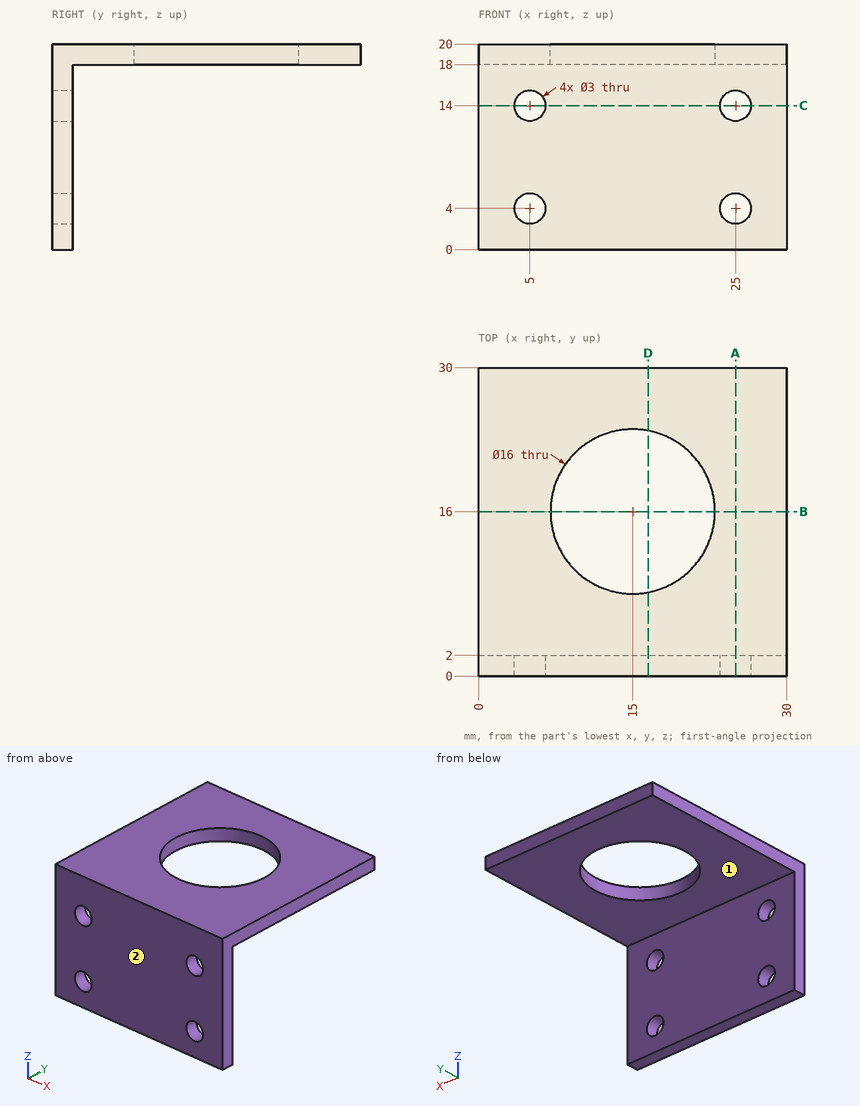
Verification items for this drawing (mm, ordinates from the low corner). A direction names the side the tool comes from. Round coordinates to 2 decimals unless told otherwise and drop trailing zeros. Write each loop counter-clockwise with the first axis right and the second up, starting at its lowest first coordinate (ties: lowest second). Pieces come first, ordered by that corner, then holes. Notation, with made-up numbers: (43.5, -4.75) - (59.5, -4.75) arc R28 ccw to (59.5, 21.25) - close; hole circle Ø4 at (22, 62). An arc over 180 degrees is marked (long way). Answer as a JSON object with one key per item and string values. Group by question number.
Q1. Section check C-C, the plane z = 14. Enter the section's corners in (x, y).
Q2. Section check A-A, the plane x = 25. Enter the section's corners in (y, z), plus the area to 3 significant figures.
Q3. Thickness scan on line 1 (X direction, y = 0.7, z = 4); line 2 (Y direction, x = 24.5, z = 2); line 3 (Z direction, x = 5.25, y = 20). Record the ranges inside material, lowest first.
Q4. Section check D-D, the plane x = 16.5. Enter the section's corners in (y, z).
Q5. Tool access check on the marked faces 1 and 2. Record the directions out of +Z, -Z, +X, -X, +Y, -Y that give a thin tool (end or side, any length) a straight path to the whole face; none if there is none.
Q6. Section check B-B, the plane y = 16. Enter the section's corners in (x, z), plus the area to 3 significant figures.
Q7. Go/stop test with flat-tipped pins: pin 1 Ø14 at (x, y) = (10, 22) entering from -Z; pin 2 Ø5 at (x, z) = (5, 14) entering from +Y. Record where each tip stops, or that it passes through.
Found:
{
 "1": {"outline": "(0, 0) - (3.5, 0) - (3.5, 2) - (0, 2) - close; (6.5, 0) - (23.5, 0) - (23.5, 2) - (6.5, 2) - close; (26.5, 0) - (30, 0) - (30, 2) - (26.5, 2) - close"},
 "2": {"outline": "(0, 0) - (2, 0) - (2, 2.5) - (0, 2.5) - close; (0, 5.5) - (2, 5.5) - (2, 12.5) - (0, 12.5) - close; (0, 15.5) - (2, 15.5) - (2, 18) - (30, 18) - (30, 20) - (0, 20) - close", "area": "84.0 mm^2"},
 "3": {"line 1": "x = 0 to 3.5, 6.5 to 23.5, 26.5 to 30", "line 2": "y = 0 to 2", "line 3": "z = 18 to 20"},
 "4": {"outline": "(0, 0) - (2, 0) - (2, 18) - (8.14, 18) - (8.14, 20) - (0, 20) - close; (23.86, 18) - (30, 18) - (30, 20) - (23.86, 20) - close"},
 "5": {"face 1": "-Z, +X, -X, +Y", "face 2": "+Z, -Z, +X, -X, -Y"},
 "6": {"outline": "(0, 18) - (7, 18) - (7, 20) - (0, 20) - close; (23, 18) - (30, 18) - (30, 20) - (23, 20) - close", "area": "28.0 mm^2"},
 "7": {"pin 1": "stops at z = 18", "pin 2": "stops at y = 2"}
}
